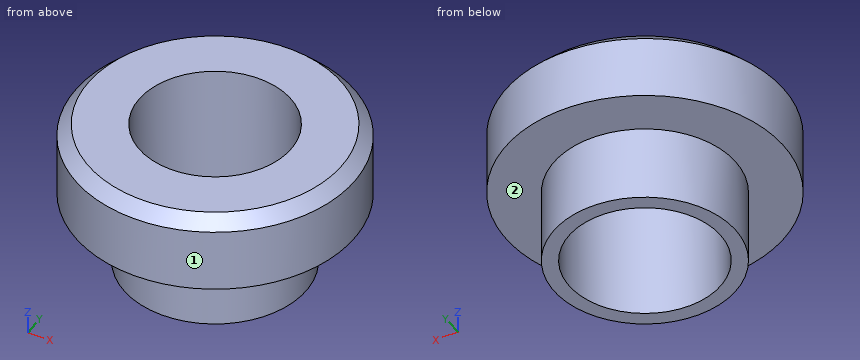
Autodesk Inventor part; units mm, degrees
ref_plane "YZ Plane" through (0, 0, 0) normal (1, 0, 0) x (0, 1, 0)
ref_plane "XZ Plane" through (0, 0, 0) normal (0, 1, 0) x (-1, 0, 0)
ref_plane "XY Plane" through (0, 0, 0) normal (0, 0, 1) x (1, 0, 0)
sketch "Эскиз1" plane through (0, 0, 0) normal (0, 1, 0) x (-1, 0, 0)
  line L0 (0, 0) -> (2.75, 0)
  line L1 (2.75, 0) -> (2.75, 1.5)
  line L2 (2.75, 1.5) -> (-2.75, 1.5)
  line L3 (-2.75, 1.5) -> (-2.75, 0)
  line L4 (-2.75, 0) -> (2.75, 0)
  line L5 (0, 0) -> (1.8, 0)
  line L6 (1.8, 0) -> (1.8, -1.5)
  line L7 (1.8, -1.5) -> (-1.8, -1.5)
  line L8 (-1.8, -1.5) -> (-1.8, 0)
  line L9 (0, 1.5) -> (1.5, 1.5)
  line L10 (1.5, 1.5) -> (1.5, -1.5)
  line L11 (0, -1.5) -> (0, 1.5)
  dimension "d0" = 2.75
  dimension "d1" = 1.5
  dimension "d2" = 5.5
  dimension "d3" = 1.8
  dimension "d4" = 1.5
  dimension "d5" = 3.6
  dimension "d6" = 1.5
revolve "Вращение1" add sketch "Эскиз1" angle 360 about axis through (0, 0, -1.5) along (0, 0, 1) contours L0 L10 L2 L1 | L6 L7 L10 L0
thread "Резьба1"
chamfer "Фаска1" distance 0.25 angle 45 1 edges at (2.75, 0, 1.5)
properties part number "soldered nut_1,5"
Source: CAD feature listing. Evaluate the final solid. Frame: model axes, mm. Face numbers are marked on the shaded views. A direction names the side the tool comes from. Give positions to 0.01 mm unless a question says otherwise; leave off trailing zeros. Loops run counter-clockwise (first coordinate to the right, second up) from the corner with the lowest first, then second, coordinate; pieces in that order, holes last. Notation, with made-up numbers: (72.25, 15.25) -> (116.25, 15.25) arc R24 ccw to (116.25, 39.25) -> close; hole circle Ø9 at (16, 47). An arc over 180 degrees is marked (long way). Use a Markdown table: item, result. Add a question column.
(1) Section query C-C (z = -0.65). Output: boundary loops of the cut face in (x, y).
(2) Ray query, line 1 (Y direction, x = 0, z = 0.3); line 2 (X direction, y = 0, z = -0.1). Return the intervals inside material, ascending.
(3) First-contact query: pin 1 Ø1 at (y, z) = (2, 0.5) entering from -X; pin 2 Ø1 at (y, z) = (1.5, -1) entering from -X. Flat tips, straight axial feed; report the tip coordinate or a pass-through.
(4) Access query for the marked faces 1 and 2. Directions: +Z, -Z, +X, -X, +Y, -Y. A direction counts if a zero-diameter tool reaches every point of the face in a straight line with its end or side. Return the directions, or none.
(5) Section query A-A (x = 0). Output: boundary loops of the cut face in (y, z), then the cut area to 3 significant figures.
(6) Section query D-D (z = 0.6). Output: boundary loops of the cut face in (x, y).
Checked values:
| question | item | result |
|---|---|---|
| 1 | outline | circle Ø3.6 at (0, 0); hole circle Ø3 at (0, 0) |
| 2 | line 1 | -2.75 to -1.5, 1.5 to 2.75 |
| 2 | line 2 | -1.8 to -1.5, 1.5 to 1.8 |
| 3 | pin 1 | x = -2.3 |
| 3 | pin 2 | x = -1.5 |
| 4 | face 1 | +Z, -Z |
| 4 | face 2 | -Z |
| 5 | outline | (-2.75, 0) -> (-1.8, 0) -> (-1.8, -1.5) -> (-1.5, -1.5) -> (-1.5, 1.5) -> (-2.5, 1.5) -> (-2.75, 1.25) -> close; (1.5, -1.5) -> (1.8, -1.5) -> (1.8, 0) -> (2.75, 0) -> (2.75, 1.25) -> (2.5, 1.5) -> (1.5, 1.5) -> close |
| 5 | area | 4.59 mm^2 |
| 6 | outline | circle Ø5.5 at (0, 0); hole circle Ø3 at (0, 0) |
